Geometry check sheet. Reference: the model listing, model coordinates, mm. A direction names the side the tool comes from. Round coordinates to 2 decimals unless told otherwise and drop trailing zeros. Order: outer loops, then holes, each group sorted by start corner. A loop starts at its lowest first (then second) coordinate and runs counter-clockwise, first axis right, second up. Notation, with made-up numbers: M 3.25,27.25 L 18.25,27.25 A29 cw 18.25,66.25 Z; hole C 69.5,16 d6. An arc over 180 degrees is marked long. Return JSON: item names as keys, results as strings. Group by question number.
```python
from build123d import *

# Parameters (mm, degrees)
SKETCH1_R           = 25
BOSS_EXTRUDE1_DEPTH = 8
SKETCH2_R           = 63
BOSS_EXTRUDE2_DEPTH = 8
SKETCH4_R           = 6
BOSS_EXTRUDE3_DEPTH = 20


with BuildPart() as part:
    # Sketch1 → Boss-Extrude1 (new body)
    with BuildSketch(Plane.XY):
        Circle(SKETCH1_R)
    extrude(amount=BOSS_EXTRUDE1_DEPTH)

    # Sketch2 → Boss-Extrude2 (add)
    with BuildSketch(Plane.XY.offset(8)):
        Circle(SKETCH2_R)
    extrude(amount=BOSS_EXTRUDE2_DEPTH)

    # Sketch4 → Boss-Extrude3 (add)
    with BuildSketch(Plane(origin=(0, 0, 8), x_dir=(-1, 0, 0), z_dir=(0, 0, -1))):
        with Locations((0, 50)):
            Circle(SKETCH4_R)
        with Locations((50, 0)):
            Circle(SKETCH4_R)
        with Locations((0, -50)):
            Circle(SKETCH4_R)
        with Locations((-50, 0)):
            Circle(SKETCH4_R)
    extrude(amount=BOSS_EXTRUDE3_DEPTH)


solid = part.part
```
Q1. Depth check by flat-ended pin: pin 1 Ø1 at (y, z) = (0.5, 3) entering from -X; pin 2 Ø6 at (y, z) = (20.5, 11.5) entering from -X; pin 3 Ø6 at (x, z) = (22.5, 5.5) entering from +Y; pin 4 Ø1.5 at (x, z) = (43, 5) entering from +Y. Enter the tip coordinate at first touch or a pass-through.
Q2. Section check A-A on x = 0. Record the cut outline in (y, z).
Q3. Release check for a two-part mould opening along X. For faces 1 (the face through (-50, 0, -12)), 2 (the face through (-8.201, 62.464, 11.944)), 3 (the face through (0, 0, 0)) record: +X half, -X half, draft (parallel to the pull), parting line (faces both ways), or undercut.
Q4. Set-up check for faces 4 (the face through (-1, 1, 16)), 5 (the face through (-44, 0, -2)): record each of +Z, -Z, +X, -X, +Y, -Y from which the full face is reachable in a straight line by a thin tool's end or side.
Q5. Section check C-C on z = 12.5. Record the cut outline in (x, y).
Q6. Section check D-D on x = 14. Record the cut outline in (y, z), plus the area to 3 significant figures.
Q7. Material ranges on line 1 along Y through (x, z) = (-50, -8.5); line 2 along Z through (x, y) = (-8.5, -57); line 3 along Y through (x, z) = (-5, 4), recorded low to high.
Geometry check:
{
 "1": {"pin 1": "stops at x = -56", "pin 2": "stops at x = -60.52", "pin 3": "stops at y = 59.45", "pin 4": "passes through"},
 "2": {"outline": "M -63,8 L -56,8 L -56,-12 L -44,-12 L -44,8 L -25,8 L -25,0 L 25,0 L 25,8 L 44,8 L 44,-12 L 56,-12 L 56,8 L 63,8 L 63,16 L -63,16 Z"},
 "3": {"face 1": "draft", "face 2": "parting line", "face 3": "undercut"},
 "4": {"face 4": "+Z, +X, -X, +Y, -Y", "face 5": "-Z"},
 "5": {"outline": "C 0,0 d126"},
 "6": {"outline": "M -61.42,8 L -20.71,8 L -20.71,0 L 20.71,0 L 20.71,8 L 61.42,8 L 61.42,16 L -61.42,16 Z", "area": "1,310 mm^2"},
 "7": {"line 1": "y = -6 to 6", "line 2": "z = 8 to 16", "line 3": "y = -53.32 to -46.68, -24.49 to 24.49, 46.68 to 53.32"}
}
